Autodesk Inventor part; units mm, degrees
ref_plane "YZ Plane" through (0, 0, 0) normal (1, 0, 0) x (0, 1, 0)
ref_plane "XZ Plane" through (0, 0, 0) normal (0, 1, 0) x (-1, 0, 0)
ref_plane "XY Plane" through (0, 0, 0) normal (0, 0, 1) x (1, 0, 0)
sketch "Sketch1" plane through (0, 0, 0) normal (0, 0, 1) x (1, 0, 0)
  line L0 (-7.6232, 4.5478) -> (61.5768, 4.5478)
  line L1 (61.5768, 4.5478) -> (61.5768, -23.9522)
  line L2 (61.5768, -23.9522) -> (-7.6232, -23.9522)
  line L3 (-7.6232, -23.9522) -> (-7.6232, 4.5478)
  line L4 (62.9768, 5.9478) -> (-9.0232, 5.9478)
  line L5 (-9.0232, 5.9478) -> (-9.0232, -25.3522)
  line L6 (-9.0232, -25.3522) -> (62.9768, -25.3522)
  line L7 (62.9768, -25.3522) -> (62.9768, 5.9478)
  point P0 (0, 0)
  dimension "d0" = 69.2
  dimension "d1" = 28.5
  dimension "d2" = 1.4
extrude "Extrusion1" add sketch "Sketch1" along normal blind 20
sketch "Sketch2" plane through (0, 0, 0) normal (0, 0, -1) x (-1, 0, 0)
  line L0 (9.0232, 5.9478) -> (9.0232, -25.3522)
  line L1 (-62.9768, 5.9478) -> (9.0232, 5.9478)
  line L2 (9.0232, -25.3522) -> (-62.9768, -25.3522)
  line L3 (-62.9768, -25.3522) -> (-62.9768, 5.9478)
  point P0 (0, 0)
extrude "Extrusion2" add sketch "Sketch2" along normal blind 1.2
sketch "Sketch3" plane through (62.9768, -25.3522, 20) normal (1, 0, 0) x (0, 0, -1)
  line L0 (20, 29.9) -> (0, 29.9)
  line L1 (20, 1.4) -> (0, 1.4)
  line L2 (20, 1.4) -> (20, 29.9)
  line L3 (20, 25.4) -> (14, 25.4)
  line L4 (14, 25.4) -> (14, 9.9)
  line L5 (14, 9.9) -> (20, 9.9)
  line L6 (20, 9.9) -> (20, 25.4)
  point P0 (20, 25.3522)
  dimension "d7" = 4.5
  dimension "d8" = 6
  dimension "d9" = 15.5
extrude "Extrusion3" cut sketch "Sketch3" against normal up to surface (1.4 mm away)
sketch "Sketch4" plane through (-9.0232, 5.9478, 20) normal (0, 1, 0) x (1, 0, 0)
  line L0 (70.6, 20) -> (70.6, 0)
  line L1 (70.6, 20) -> (1.4, 20)
  line L2 (68, 18.9) -> (57, 18.9)
  line L3 (57, 18.9) -> (57, 13.5)
  line L4 (57, 13.5) -> (68, 13.5)
  line L5 (68, 13.5) -> (68, 18.9)
  point P0 (9.0232, 20)
  dimension "d12" = 11
  dimension "d13" = 2.6
  dimension "d14" = 1.1
  dimension "d15" = 5.4
extrude "Extrusion4" cut sketch "Sketch4" against normal up to surface (1.4 mm away)
chamfer "Chamfer1" distance 2 angle 45 1 edges at (62.2768, -15.4522, 6)
chamfer "Chamfer2" distance 2 angle 45 1 edges at (62.2768, 0.0478, 6)
sketch "Sketch5" plane through (-9.0232, 5.9478, 20) normal (0, 1, 0) x (1, 0, 0)
  line L0 (1.4, 20) -> (1.4, 0)
  line L1 (70.6, 20) -> (1.4, 20)
  line L2 (13.1, 16) -> (28.6, 16)
  line L3 (28.6, 16) -> (28.6, 9.8)
  line L4 (28.6, 9.8) -> (13.1, 9.8)
  line L5 (13.1, 9.8) -> (13.1, 16)
  point P0 (9.0232, 20)
  dimension "d24" = 4
  dimension "d25" = 6.2
  dimension "d26" = 15.5
  dimension "d27" = 11.7
extrude "Extrusion5" cut sketch "Sketch5" against normal up to surface (1.4 mm away)
chamfer "Chamfer3" distance 2 angle 45 2 edges at (4.0768, 5.2478, 10.2) (19.5768, 5.2478, 10.2)
sketch "Sketch6" plane through (-9.0232, -25.3522, 20) normal (-1, 0, 0) x (0, 0, 1)
  line L0 (-20, 1.4) -> (0, 1.4)
  line L1 (-20, 29.9) -> (-20, 1.4)
  line L2 (-14.8, 6.4) -> (-9.6, 6.4)
  line L3 (-9.6, 6.4) -> (-9.6, 16.9)
  line L4 (-9.6, 16.9) -> (-14.8, 16.9)
  line L5 (-14.8, 16.9) -> (-14.8, 6.4)
  point P0 (-20, 25.3522)
  dimension "d33" = 5
  dimension "d34" = 10.5
  dimension "d35" = 5.2
  dimension "d36" = 5.2
extrude "Extrusion6" cut sketch "Sketch6" against normal up to surface (1.4 mm away)
sketch "Sketch8" plane through (62.9768, -25.3522, 20) normal (1, 0, 0) x (0, 0, -1)
  line L0 (16, 9.9) -> (20, 9.9)
  line L1 (0, 29.9) -> (0, 1.4)
  line L2 (16, 9.9) -> (0, 9.9)
  line L3 (0, 9.9) -> (0, 25.3522)
  line L4 (0, 25.3522) -> (16, 25.3522)
  line L5 (16, 25.3522) -> (16, 9.9)
  point P0 (20, 25.3522)
extrude "Extrusion7" cut sketch "Sketch8" against normal up to surface (1.4 mm away)
sketch "Sketch9" plane through (-7.6232, 4.5478, 20) normal (0, -1, 0) x (1, 0, 0)
  line L0 (27.2, -11.8) -> (25.2, -9.8)
  line L1 (13.7, -9.8) -> (11.7, -11.8)
  line L2 (0, 0) -> (69.2, 0)
  line L3 (11.7, -11.8) -> (27.2, -11.8)
  line L4 (27.2, -11.8) -> (27.2, 0)
  line L5 (27.2, 0) -> (11.7, 0)
  line L6 (11.7, 0) -> (11.7, -11.8)
  line L7 (55.6, -13.5) -> (66.6, -13.5)
  line L8 (55.6, -13.5) -> (66.6, -13.5)
  line L9 (66.6, -13.5) -> (66.6, 0)
  line L10 (66.6, 0) -> (55.6, 0)
  line L11 (55.6, 0) -> (55.6, -13.5)
  point P0 (7.6232, -20)
extrude "Extrusion8" cut sketch "Sketch9" against normal up to surface (1.4 mm away)
sketch "Sketch10" plane through (-9.0232, -25.3522, 20) normal (-1, 0, 0) x (0, 0, 1)
  line L0 (-9.6, 16.9) -> (-9.6, 6.4)
  line L1 (0, 1.4) -> (0, 29.9)
  line L2 (-9.6, 6.4) -> (0, 6.4)
  line L3 (0, 6.4) -> (0, 16.9)
  line L4 (0, 16.9) -> (-9.6, 16.9)
  line L5 (-9.6, 16.9) -> (-9.6, 6.4)
  point P0 (-20, 25.3522)
extrude "Extrusion9" cut sketch "Sketch10" against normal up to surface (1.4 mm away)
properties part number "PlutoIIxHDMI"
The listing builds one solid part. Answer for the finished solid, in the listing's coordinates (mm). A direction names the side the tool comes from. Coordinates: 2 decimals unless noted, no trailing zeros. Write each loop counter-clockwise with the first axis right and the second up, starting at its lowest first coordinate (ties: lowest second). Pieces come first, ordered by that corner, then holes. Notation, with made-up numbers: (-38.75, -17.75) - (-23.75, -17.75) arc R35 cw to (-23.75, 17.25) - close; hole circle Ø1 at (-39.75, 73.25). An arc over 180 degrees is marked (long way). Return JSON: item names as keys, results as strings. Group by question number.
1. Determine the mould class of faces 4 (the flat face through (26, -25.352, 9)), 5 (the flat face through (47.977, 5, 11)), 6 (the flat face through (61.577, -20, 10)) for opening direction Y: released by +Y, released by -Y, zero draft, split by the parting line, or undercut.
2. A cutting plane is placed at B-B, the plane x = 57.5. Determine the outline of the cut face in (y, z), plus the area to 3 significant figures.
3. A cutting plane is placed at D-D, the plane y = -3. Determine the outline of the cut face in (x, z), plus the area to 3 significant figures.
4. Given pin 1 (1.5 mm diameter, centred on y = -1, z = 13, fed in from +X); pin 2 (1.5 mm diameter, centred on x = 9, y = -17, fed in from +Z), each flat-ended and moving along its own axis, determine where each tip first touches the part or whether it passes through.
5. Which of the six approach directions +Z, -Z, +X, -X, +Y, -Y give full straight-line access (tool end or side, diameter ignored) to faces 1 (the flat face through (26, 4.548, 10)), 2 (the flat face through (-8, -18.952, 12)), 3 (the flat face through (4.077, 5, 12))?
6. Straight lines are drawn through the part: L1, parallel to Y at x = 29.5, z = 18.5; L2, parallel to X at y = -19, z = 4.75; L3, parallel to X at y = -7, z = 11.5. For each, find the intervals that lie inside material, in ascending order.
7. A cutting plane is placed at A-A, the plane z = 2.25. Determine the outline of the cut face in (x, y), plus the area to 3 significant figures.
8. A cutting plane is placed at C-C, the plane z = 18. Determine the outline of the cut face in (x, y).
Ans:
{
 "1": {"face 4": "released by -Y", "face 5": "zero draft", "face 6": "undercut"},
 "2": {"outline": "(-25.35, -1.2) - (5.95, -1.2) - (5.95, 1.1) - (4.55, 1.1) - (4.55, 0) - (-23.95, 0) - (-23.95, 20) - (-25.35, 20) - close", "area": "67.1 mm²"},
 "3": {"outline": "(-9.02, -1.2) - (62.98, -1.2) - (62.98, 0) - (-7.62, 0) - (-7.62, 20) - (-9.02, 20) - close", "area": "114 mm²"},
 "4": {"pin 1": "x = -7.62", "pin 2": "z = 0"},
 "5": {"face 1": "+Z", "face 2": "+Z, -X", "face 3": "+Z, +Y"},
 "6": {"L1": "-25.35 to -23.95, 4.55 to 5.95", "L2": "-9.02 to -7.62, 61.58 to 62.98", "L3": "-9.02 to -7.62"},
 "7": {"outline": "(-9.02, -25.35) - (62.98, -25.35) - (62.98, -15.45) - (61.58, -15.45) - (61.58, -23.95) - (-7.62, -23.95) - (-7.62, 4.55) - (47.98, 4.55) - (47.98, 5.95) - (-9.02, 5.95) - close; (58.98, 4.55) - (61.58, 4.55) - (61.58, 0.05) - (62.98, 0.05) - (62.98, 5.95) - (58.98, 5.95) - close", "area": "244 mm²"},
 "8": {"outline": "(-9.02, -25.35) - (62.98, -25.35) - (62.98, -15.45) - (61.58, -15.45) - (61.58, -23.95) - (-7.62, -23.95) - (-7.62, -18.95) - (-9.02, -18.95) - close; (-9.02, -8.45) - (-7.62, -8.45) - (-7.62, 4.55) - (4.08, 4.55) - (4.08, 5.95) - (-9.02, 5.95) - close; (19.58, 4.55) - (47.98, 4.55) - (47.98, 5.95) - (19.58, 5.95) - close; (58.98, 4.55) - (61.58, 4.55) - (61.58, 0) - (62.98, 0) - (62.98, 5.95) - (58.98, 5.95) - close"}
}
